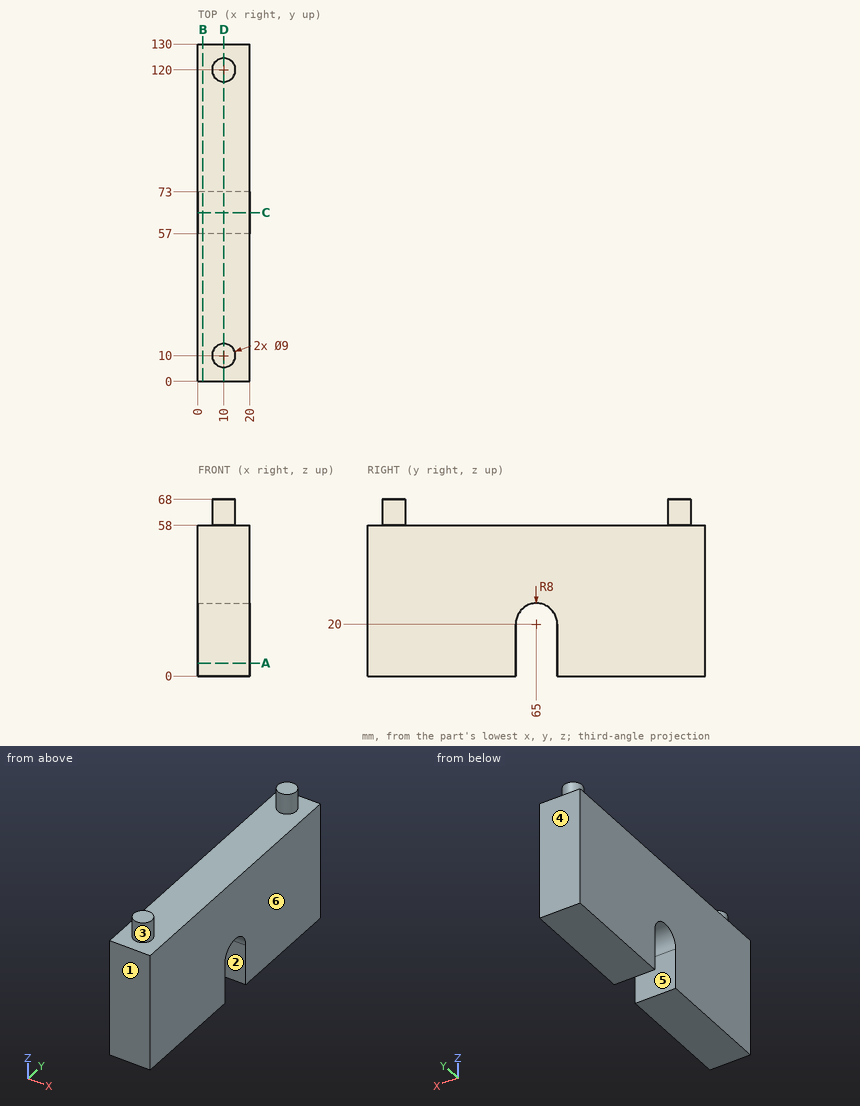
Geometry check sheet. Reference: drawing and pictorial views, mm from the part's lowest x, y, z. A direction names the side the tool comes from. Coordinates: 2 decimals unless noted, no trailing zeros. Write each loop counter-clockwise with the first axis right and the second up, starting at its lowest first coordinate (ties: lowest second). Pieces come first, ordered by that corner, then holes. Notation, with made-up numbers: (52, 12.25) - (85, 12.25) arc R12 cw to (85, 20.25) - close; hole circle Ø4 at (27.25, -7). An arc over 180 degrees is marked (long way). One line per question, with ' | ' between items. Start each with the question number.
1. Section check B-B (x = 2). Enter the section's corners in (y, z).
2. Draft check along Y on the marked faces 4, 5 and 6. Enter one of: released by +Y, released by -Y, zero draft, split by the parting line, or undercut.
3. Section check A-A (z = 5). Enter the section's corners in (x, y).
4. Access from +Z, -Z, +X, -X, +Y, -Y to the whole of each face (thin tool, end or side, straight path). Record for the marked faces 1, 2 and 3.
5. Section check D-D (x = 10). Enter the section's corners in (y, z).
6. Material ranges on line 1 along Y through (x, z) = (3, 14); line 2 along Z through (x, y) = (3.75, 16.5); line 3 along Y through (x, z) = (19.25, 25) (3 decimals), recorded low to high.
7. Gauge pin test, flat end, axial feed: P1, Ø1.5, axis at x = 15, y = 67, coming from the +Z side. Record the tip position at first contact, or that the pin passes through.
8. Section check C-C (y = 65). Enter the section's corners in (x, z), plus the area to 3 significant figures.
Computed values:
1) outline: (0, 0) - (57, 0) - (57, 20) arc R8 cw to (73, 20) - (73, 0) - (130, 0) - (130, 58) - (0, 58) - close
2) face 4: released by +Y | face 5: undercut | face 6: zero draft
3) outline: (0, 0) - (20, 0) - (20, 57) - (0, 57) - close; (0, 73) - (20, 73) - (20, 130) - (0, 130) - close
4) face 1: +Z, -Z, +X, -X, -Y | face 2: -Z, +X, -X | face 3: +Z
5) outline: (0, 0) - (57, 0) - (57, 20) arc R8 cw to (73, 20) - (73, 0) - (130, 0) - (130, 58) - (124.5, 58) - (124.5, 68) - (115.5, 68) - (115.5, 58) - (14.5, 58) - (14.5, 68) - (5.5, 68) - (5.5, 58) - (0, 58) - close
6) line 1: 0 to 57, 73 to 130 | line 2: 0 to 58 | line 3: 0 to 58.755, 71.245 to 130
7) P1: z = 58
8) outline: (0, 28) - (20, 28) - (20, 58) - (0, 58) - close | area: 600 mm²
